Autodesk Inventor part; units mm, degrees
ref_plane "YZ Plane" through (0, 0, 0) normal (1, 0, 0) x (0, 1, 0)
ref_plane "XZ Plane" through (0, 0, 0) normal (0, 1, 0) x (-1, 0, 0)
ref_plane "XY Plane" through (0, 0, 0) normal (0, 0, 1) x (1, 0, 0)
sketch "Boceto1" plane through (0, 0, 0) normal (0, 0, 1) x (1, 0, 0)
  circle A0 centre (0, 0) radius 5
  dimension "d0" = 10
extrude "Extrusión1" add sketch "Boceto1" along normal blind 30
sketch "Boceto2" plane through (0, 0, 30) normal (0, 0, 1) x (1, 0, 0)
  circle A0 centre (0, 0) radius 5
  circle A1 centre (0, 0) radius 2.9
  dimension "d3" = 5.8
extrude "Extrusión2" cut sketch "Boceto2" against normal blind 25
fillet "Empalme1" radius 0.5 3 edges at (-2.9, 0, 30) (-5, 0, 5) (-5, 0, 0)
properties part number "pern frontissa"
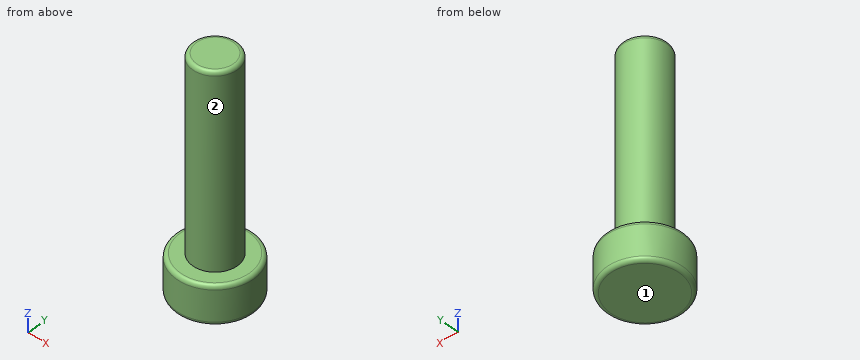
Here's how the part is built. I have some questions about the finished solid (model axes, mm). Face numbers are marked on the shaded views. A direction names the side the tool comes from. Round coordinates to 2 decimals unless told otherwise and drop trailing zeros. Loops run counter-clockwise (first coordinate to the right, second up) from the corner with the lowest first, then second, coordinate; pieces in that order, holes last.
1. If we section it at C-C on z = 26.5: Write out the boundary of the cut face in (x, y).
Answer list:
outline: circle Ø5.8 at (0, 0)
2. For P1, Ø1.5, axis at y = -1.5, z = 18.5, coming from the +X side; P2, Ø6, axis at x = -3.5, z = 7, coming from the -Y side; P3, Ø1, axis at y = -1.5, z = 18, coming from the +X side, each with a flat end and sliding along its axis, tell me the tip position at first contact or that it passes through.
Answer list:
P1: stops at x = 2.8
P2: stops at y = -4.7
P3: stops at x = 2.72
3. Which directions (+Z, -Z, +X, -X, +Y, -Y) give clear straight access to the entire face, cutting with the end or side of a thin tool? Please do the marked faces 1 and 2.
Answer list:
face 1: -Z, +X, -X, +Y, -Y
face 2: +Z
4. If we section it at A-A on x = 0: Write out the boundary of the cut face in (y, z).
Answer list:
outline: (-5, 0.5) arc R0.5 ccw to (-4.5, 0) - (4.5, 0) arc R0.5 ccw to (5, 0.5) - (5, 4.5) arc R0.5 ccw to (4.5, 5) - (2.9, 5) - (2.9, 29.5) arc R0.5 ccw to (2.4, 30) - (-2.4, 30) arc R0.5 ccw to (-2.9, 29.5) - (-2.9, 5) - (-4.5, 5) arc R0.5 ccw to (-5, 4.5) - close
5. If I drill on line 1 along Z through (x, y) = (4, -1); line 2 along Y through (x, z) = (-1.5, 11); line 3 along X through (y, z) = (0.25, 27.5), over which ranges is the centre line in solid material (lowest first)?
Answer list:
line 1: z = 0 to 5
line 2: y = -2.48 to 2.48
line 3: x = -2.89 to 2.89
